Autodesk Inventor part; units mm, degrees
ref_plane "YZ Plane" through (0, 0, 0) normal (1, 0, 0) x (0, 1, 0)
ref_plane "XZ Plane" through (0, 0, 0) normal (0, 1, 0) x (-1, 0, 0)
ref_plane "XY Plane" through (0, 0, 0) normal (0, 0, 1) x (1, 0, 0)
sketch "Boceto1" plane through (0, 0, 0) normal (0, 0, 1) x (1, 0, 0)
  circle A0 centre (0, 0) radius 6
  circle A1 centre (0, 0) radius 2.5
extrude "Extrusión1" add sketch "Boceto1" along normal blind 4
sketch "Boceto2" plane through (0, 0, 4) normal (0, 0, 1) x (1, 0, 0)
  circle A0 centre (0, 0) radius 6
  circle A1 centre (0, 0) radius 5
fillet "Empalme1" radius 0.3 2 edges at (-2.5, 0, 4) (-2.5, 0, 0)
extrude "Extrusión3" cut sketch "Boceto2" against normal blind 3
chamfer "Chaflán2" distance 0.3 angle 45 2 edges at (-5, 0, 4) (-6, 0, 1)
properties part number "cojinete polea x"
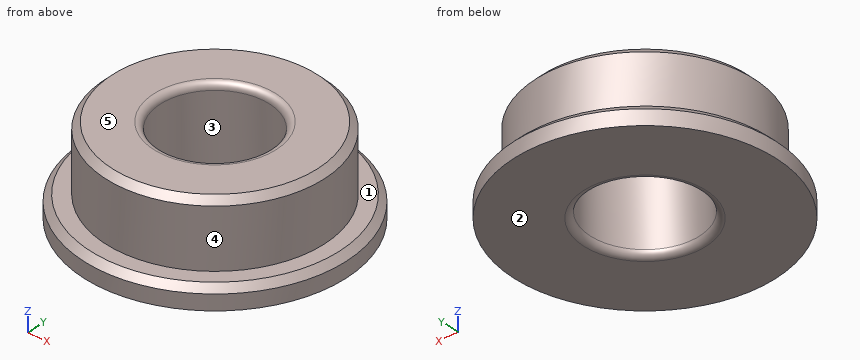
Part model, mm, in its own coordinate system. Face numbers are marked on the shaded views. A direction names the side the tool comes from. Round coordinates to 2 decimals unless told otherwise and drop trailing zeros. Order: outer loops, then holes, each group sorted by start corner. A loop starts at its lowest first (then second) coordinate and runs counter-clockwise, first axis right, second up. Notation, with made-up numbers: M 79,-2.75 L 111,-2.75 A24 cw 111,11.25 Z; hole C 61.25,65.25 d9. An arc over 180 degrees is marked long. Answer in a Markdown table with one row per item. Add a question column.
Q1. Cut at A-A on y = 0. Give the cut face in (x, z).
Q2. 3-axis set-ups, long thin cutter, end or side, ignore diameter. For the marked faces 1 and 2: which of +Z, -Z, +X, -X, +Y, -Y reach the whole face in a straight line?
Q3. Pin check, flat tips, straight feed: pin 1 (1.5 mm diameter, centred on y = -1, z = 2, fed in from +X); pin 2 (1 mm diameter, centred on x = 1.5, z = 3, fed in from +Y). Stop position of each tip, or through.
Q4. Cut at C-C on z = 1.7. Give the cut face in (x, y), and give its area (3 significant figures).
Q5. Mould opens along X. For the marked faces 3, 4 and 5 say: +X half, -X half, draft (parallel to the pull), parting line (faces both ways), or undercut.
Q6. Wall check: L1, parallel to Y at x = 0, z = 3.35; L2, parallel to Z at x = 4.5, y = 2.5; L3, parallel to X at y = -0.75, z = 3.35. Give the ranges that are in metal, low to high. Write a range as from..to.
Established:
| question | item | result |
|---|---|---|
| 1 | outline | M -6,0 L -2.8,0 A0.3 ccw -2.5,0.3 L -2.5,3.7 A0.3 ccw -2.8,4 L -4.7,4 L -5,3.7 L -5,1 L -5.7,1 L -6,0.7 Z; M 2.5,0.3 A0.3 ccw 2.8,0 L 6,0 L 6,0.7 L 5.7,1 L 5,1 L 5,3.7 L 4.7,4 L 2.8,4 A0.3 ccw 2.5,3.7 Z |
| 2 | face 1 | +Z |
| 2 | face 2 | -Z, +X, -X, +Y, -Y |
| 3 | pin 1 | stops at x = 4.99 |
| 3 | pin 2 | stops at y = 4.9 |
| 4 | outline | C 0,0 d10; hole C 0,0 d5 |
| 4 | area | 58.9 mm2 |
| 5 | face 3 | undercut |
| 5 | face 4 | parting line |
| 5 | face 5 | draft |
| 6 | L1 | y = -5..-2.5, 2.5..5 |
| 6 | L2 | z = 0..1 |
| 6 | L3 | x = -4.94..-2.38, 2.38..4.94 |
